Read the model definition and answer for the solid it produces. Units are mm, in the model's axes. Coordinates: 2 decimals unless noted, no trailing zeros. Loops run counter-clockwise (first coordinate to the right, second up) from the corner with the lowest first, then second, coordinate; pieces in that order, holes last. Notation, with made-up numbers: (5.25, 75) -> (62.25, 75) arc R16 cw to (62.25, 103) -> close; hole circle Ø1 at (-30, 69). An arc over 180 degrees is marked (long way). Answer as CSV lines item,"result".
```python
from build123d import *

# Parameters (mm, degrees)
SKETCH2_R           = 3.175
SKETCH2_R_2         = 1.5875
SKETCH2_R_3         = 4.7625
SKETCH2_R_4         = 1.524
BOSS_EXTRUDE2_DEPTH = 2.9718
CUT_EXTRUDE1_DEPTH  = 72.903419609
FILLET1_R           = 2.54


with BuildPart() as part:
    # Sketch2 → Boss-Extrude2 (new body)
    # profile 1 of 10: a face of its own
    with BuildSketch(Plane(origin=(0, 0, 0), x_dir=(1, 0, 0), z_dir=(0, 1, 0))):
        with BuildLine():
            ThreePointArc((4.7625, -46.825), (3.424205755, -50.135018308), (0.161462226, -51.5847622))
            Line((0.161462226, -51.5847622), (46.932641484, -49.9981748))
            ThreePointArc((46.932641484, -49.9981748), (44.542196163, -44.618321128), (50, -46.825))
            Line((50, -46.825), (50, 46.825))
            ThreePointArc((50, 46.825), (44.57993597, 44.57993597), (46.825, 50))
            Line((46.825, 50), (-46.825, 50))
            ThreePointArc((-46.825, 50), (-44.57993597, 49.07006403), (-43.65, 46.825))
            ThreePointArc((-43.65, 46.825), (-46.825, 43.65), (-50, 46.825))
            Line((-50, 46.825), (-50, -46.825))
            ThreePointArc((-50, -46.825), (-46.825, -43.65), (-43.65, -46.825))
            ThreePointArc((-43.65, -46.825), (-44.618321128, -49.107803837), (-46.932641484, -49.9981748))
            Line((-46.932641484, -49.9981748), (-0.161462226, -51.5847622))
            ThreePointArc((-0.161462226, -51.5847622), (-3.310018308, -43.400794245), (4.7625, -46.825))
        make_face()
        with Locations((-46.026877933, 11.948327334)):
            Circle(SKETCH2_R, mode=Mode.SUBTRACT)
        with Locations((-43.813122067, 37.251672666)):
            Circle(SKETCH2_R, mode=Mode.SUBTRACT)
        with Locations((46.026877933, 11.948327334)):
            Circle(SKETCH2_R, mode=Mode.SUBTRACT)
        with Locations((43.813122067, 37.251672666)):
            Circle(SKETCH2_R, mode=Mode.SUBTRACT)
    # profile 2 of 10: a face of its own
    with BuildSketch(Plane(origin=(0, 0, 0), x_dir=(1, 0, 0), z_dir=(0, 1, 0))):
        with Locations((-46.825, -46.825)):
            Circle(SKETCH2_R)
        with Locations(Location((-46.825, -46.825, 0), (0, 0, 270))):
            Circle(SKETCH2_R_2, mode=Mode.SUBTRACT)
    # profile 3 of 10: a face of its own
    with BuildSketch(Plane(origin=(0, 0, 0), x_dir=(1, 0, 0), z_dir=(0, 1, 0))):
        with Locations((0, -46.825)):
            Circle(SKETCH2_R_3)
        with Locations(Location((0, -46.825, 0), (0, 0, 270))):
            Circle(SKETCH2_R_2, mode=Mode.SUBTRACT)
    # profile 4 of 10: a face of its own
    with BuildSketch(Plane(origin=(0, 0, 0), x_dir=(1, 0, 0), z_dir=(0, 1, 0))):
        with Locations((46.825, -46.825)):
            Circle(SKETCH2_R)
        with Locations(Location((46.825, -46.825, 0), (0, 0, 270))):
            Circle(SKETCH2_R_2, mode=Mode.SUBTRACT)
    # profile 5 of 10: a face of its own
    with BuildSketch(Plane(origin=(0, 0, 0), x_dir=(1, 0, 0), z_dir=(0, 1, 0))):
        with Locations((46.026877933, 11.948327334)):
            Circle(SKETCH2_R)
        with Locations(Location((46.026877933, 11.948327334, 0), (0, 0, 270))):
            Circle(SKETCH2_R_4, mode=Mode.SUBTRACT)
    # profile 6 of 10: a face of its own
    with BuildSketch(Plane(origin=(0, 0, 0), x_dir=(1, 0, 0), z_dir=(0, 1, 0))):
        with Locations((43.813122067, 37.251672666)):
            Circle(SKETCH2_R)
        with Locations(Location((43.813122067, 37.251672666, 0), (0, 0, 270))):
            Circle(SKETCH2_R_4, mode=Mode.SUBTRACT)
    # profile 7 of 10: a face of its own
    with BuildSketch(Plane(origin=(0, 0, 0), x_dir=(1, 0, 0), z_dir=(0, 1, 0))):
        with Locations((46.825, 46.825)):
            Circle(SKETCH2_R)
        with Locations(Location((46.825, 46.825, 0), (0, 0, 270))):
            Circle(SKETCH2_R_2, mode=Mode.SUBTRACT)
    # profile 8 of 10: a face of its own
    with BuildSketch(Plane(origin=(0, 0, 0), x_dir=(1, 0, 0), z_dir=(0, 1, 0))):
        with Locations((-43.813122067, 37.251672666)):
            Circle(SKETCH2_R)
        with Locations(Location((-43.813122067, 37.251672666, 0), (0, 0, 270))):
            Circle(SKETCH2_R_4, mode=Mode.SUBTRACT)
    # profile 9 of 10: a face of its own
    with BuildSketch(Plane(origin=(0, 0, 0), x_dir=(1, 0, 0), z_dir=(0, 1, 0))):
        with Locations((-46.825, 46.825)):
            Circle(SKETCH2_R)
        with Locations(Location((-46.825, 46.825, 0), (0, 0, 270))):
            Circle(SKETCH2_R_2, mode=Mode.SUBTRACT)
    # profile 10 of 10: a face of its own
    with BuildSketch(Plane(origin=(0, 0, 0), x_dir=(1, 0, 0), z_dir=(0, 1, 0))):
        with Locations((-46.026877933, 11.948327334)):
            Circle(SKETCH2_R)
        with Locations(Location((-46.026877933, 11.948327334, 0), (0, 0, 270))):
            Circle(SKETCH2_R_4, mode=Mode.SUBTRACT)
    extrude(amount=BOSS_EXTRUDE2_DEPTH)

    # Sketch3 → Cut-Extrude1 (cut, through all)
    with BuildSketch(Plane(origin=(0, 0, 0), x_dir=(1, 0, 0), z_dir=(0, 1, 0))):
        Polygon((-5.215323358, -44.285), (-43.584931126, 4.710491728), (-44.250273466, -44.285), align=None)
        Polygon((-2.54, 9.408327334), (-40.811554575, 9.408327334), (-2.54, -39.461956848), align=None)
        Polygon((2.54, -39.461956848), (40.811554575, 9.408327334), (2.54, 9.408327334), align=None)
        Polygon((44.250273466, -44.285), (43.584931126, 4.710491728), (5.215323358, -44.285), align=None)
        with BuildLine():
            Line((43.363147562, 44.285), (7.557737131, 44.285))
            Line((7.557737131, 44.285), (42.997535117, 17.43064252))
            Line((42.997535117, 17.43064252), (41.448819224, 35.132546179))
            ThreePointArc((41.448819224, 35.132546179), (40.65688527, 37.596338128), (41.961912119, 39.831139031))
            Line((41.961912119, 39.831139031), (43.363147562, 44.285))
        make_face()
        Polygon((38.469140802, 14.488327334), (2.54, 41.713482269), (2.54, 14.488327334), align=None)
        Polygon((-2.54, 14.488327334), (-2.54, 41.713482269), (-38.469140802, 14.488327334), align=None)
        with BuildLine():
            Line((-42.997535117, 17.43064252), (-7.557737131, 44.285))
            Line((-7.557737131, 44.285), (-43.363147562, 44.285))
            Line((-43.363147562, 44.285), (-41.961912119, 39.831139031))
            ThreePointArc((-41.961912119, 39.831139031), (-40.988390524, 38.70133356), (-40.638122067, 37.251672666))
            ThreePointArc((-40.638122067, 37.251672666), (-40.847714294, 36.117220491), (-41.448819224, 35.132546179))
            Line((-41.448819224, 35.132546179), (-42.997535117, 17.43064252))
        make_face()
    extrude(amount=CUT_EXTRUDE1_DEPTH, mode=Mode.SUBTRACT)

    # Fillet1
    fillet1_edges = [part.edges().sort_by_distance(p)[0] for p in [
        (41.448819224, 1.4859, -35.132546179),
        (41.961912119, 1.4859, -39.831139031),
        (43.363147562, 1.4859, -44.285),
        (7.557737131, 1.4859, -44.285),
        (42.997535117, 1.4859, -17.43064252),
        (5.215323358, 1.4859, 44.285),
        (44.250273466, 1.4859, 44.285),
        (43.584931126, 1.4859, -4.710491728),
        (40.811554575, 1.4859, -9.408327334),
        (2.54, 1.4859, -9.408327334),
        (2.54, 1.4859, 39.461956848),
        (-2.54, 1.4859, 39.461956848),
        (-2.54, 1.4859, -9.408327334),
        (-40.811554575, 1.4859, -9.408327334),
        (-41.961912119, 1.4859, -39.831139031),
        (-41.448819224, 1.4859, -35.132546179),
        (-42.997535117, 1.4859, -17.43064252),
        (-7.557737131, 1.4859, -44.285),
        (-43.363147562, 1.4859, -44.285),
        (-2.54, 1.4859, -41.713482269),
        (-38.469140802, 1.4859, -14.488327334),
        (-2.54, 1.4859, -14.488327334),
        (2.54, 1.4859, -41.713482269),
        (2.54, 1.4859, -14.488327334),
        (38.469140802, 1.4859, -14.488327334),
        (-43.584931126, 1.4859, -4.710491728),
        (-44.250273466, 1.4859, 44.285),
        (-5.215323358, 1.4859, 44.285),
    ]]
    fillet(fillet1_edges, radius=FILLET1_R)


solid = part.part
```
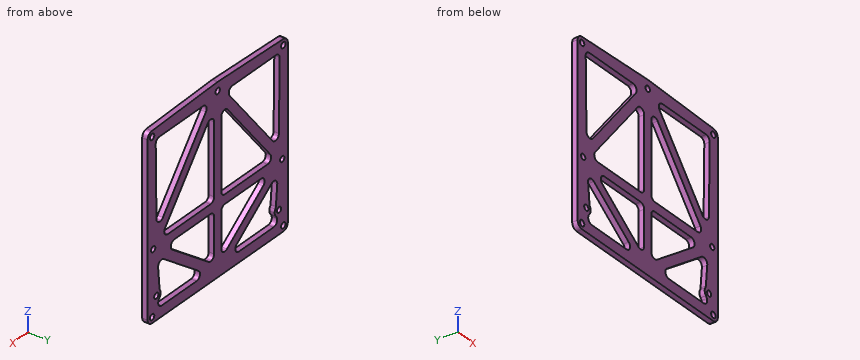
Q1. A cutting plane is placed at A-A, the plane z = 11.5. Write down the section's boundary in (x, y), and give its area (3 significant figures).
Results:
outline,"(-50, 0) -> (-43.81, 0) -> (-43.81, 2.97) -> (-50, 2.97) -> close; (-30.89, 0) -> (-24.44, 0) -> (-24.44, 2.97) -> (-30.89, 2.97) -> close; (-2.54, 0) -> (2.54, 0) -> (2.54, 2.97) -> (-2.54, 2.97) -> close; (24.44, 0) -> (30.89, 0) -> (30.89, 2.97) -> (24.44, 2.97) -> close; (43.81, 0) -> (50, 0) -> (50, 2.97) -> (43.81, 2.97) -> close"
area,"90.3 mm²"
Q2. A cutting plane is placed at B-B, the plane z = 36.5. Write down the section's boundary in (x, y).
Results:
outline,"(-50, 0) -> (-44.14, 0) -> (-44.14, 2.97) -> (-50, 2.97) -> close; (-11.31, 0) -> (11.31, 0) -> (11.31, 2.97) -> (-11.31, 2.97) -> close; (44.14, 0) -> (50, 0) -> (50, 2.97) -> (44.14, 2.97) -> close"
Q3. Find the intervals of material crossed by probe 1 along X at (y, z) = (2.65, 29.5); probe 2 along X at (y, z) = (2.05, -28); probe 3 along Z at (x, y) = (36.5, 2.6) (1 decimal), in increasing order. Write a range as [from, to].
Results:
probe 1,"x = [-50, -44.05], [-16.79, -10.34], [-2.54, 2.54], [10.34, 16.79], [44.05, 50]"
probe 2,"x = [-50, -42.07], [-29.05, -20.64], [-2.54, 2.54], [20.64, 29.05], [42.07, 50]"
probe 3,"z = [-50, -44.3], [-22.4, -9.2], [-3.9, 4.3], [44.3, 50.4]"
Q4. A cutting plane is placed at D-D, the plane y = 2.25. Give the number of separate pieces and of enclosed holes in the cut face, and give its area (3 significant figures).
Results:
separate pieces,"1"
enclosed holes,"17"
area,"4,480 mm²"
Q5. Given pin 1 Ø1.5 at (x, y) = (-32.5, 2) entering from +Z; pin 2 Ø4 at (x, z) = (-46.03, -11.95) entering from -Y; pin 3 Ø6 at (x, z) = (-15, 15.5) entering from +Y; pin 4 Ø1.5 at (x, y) = (17, 1.5) entering from +Z, each flat-ended and moving along its own axis, determine where each tip first touches the part or whether it passes through.
Results:
pin 1,"stops at z = 50.51"
pin 2,"stops at y = 0"
pin 3,"passes through"
pin 4,"stops at z = 51.04"
Q6. A cutting plane is placed at C-C, the plane z = -3. Write down the section's boundary in (x, y), and give its area (3 significant figures).
Results:
outline,"(-50, 0) -> (-35.79, 0) -> (-35.79, 2.97) -> (-50, 2.97) -> close; (-2.54, 0) -> (2.54, 0) -> (2.54, 2.97) -> (-2.54, 2.97) -> close; (35.79, 0) -> (50, 0) -> (50, 2.97) -> (35.79, 2.97) -> close"
area,"99.5 mm²"
